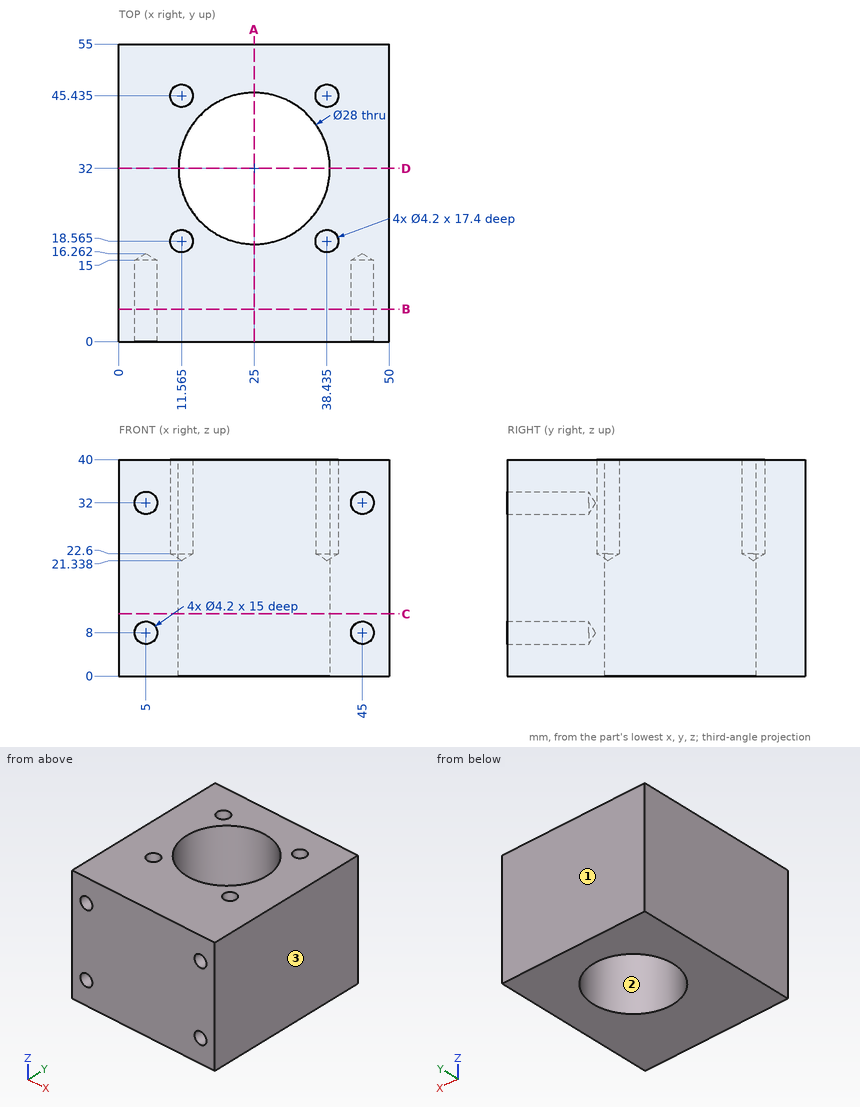
Print and shaded views of the part. All mm, measured from the part's lowest x, y and z. Give positions to 0.01 mm unless a question says otherwise; leave off trailing zeros. Loops run counter-clockwise (first coordinate to the right, second up) from the corner with the lowest first, then second, coordinate; pieces in that order, holes last.
1) Saw through at C-C (z = 11.5). Write the cut outline in (x, y), plus the area to 3 significant figures.
2) Saw through at A-A (x = 25). Write the cut outline in (y, z).
3) Saw through at D-D (y = 32). Write the cut outline in (x, z), plus the area to 3 significant figures.
4) Saw through at B-B (y = 6). Write the cut outline in (x, z), plus the area to 3 significant figures.
5) Wall check: line 1 (Z direction, x = 45, y = 8); line 2 (X direction, y = 17, z = 26) (1 decimal); line 3 (Y direction, x = 12.5, z = 37.5) (1 decimal). Give the ranges that are in metal, low to high.
6) Flat gauge pins, fed straight in: pin 1 Ø4 at (x, z) = (5, 8) entering from -Y; pin 2 Ø3.5 at (x, z) = (5, 32) entering from -Y. Where does each tip first touch, or does it go through?
7) Pull direction X, two halves, no side cores. Call the marked faces 1, 2 and 3: +X half, -X half, draft (parallel to the pull), parting line (faces both ways), or undercut.
Answer block:
1. outline: (0, 0) - (50, 0) - (50, 55) - (0, 55) - close; hole circle Ø28 at (25, 32)
1. area: 2,130 mm2
2. outline: (0, 0) - (18, 0) - (18, 40) - (0, 40) - close; (46, 0) - (55, 0) - (55, 40) - (46, 40) - close
3. outline: (0, 0) - (11, 0) - (11, 40) - (0, 40) - close; (39, 0) - (50, 0) - (50, 40) - (39, 40) - close
3. area: 880 mm2
4. outline: (0, 0) - (50, 0) - (50, 40) - (0, 40) - close; hole circle Ø4.2 at (5, 8); hole circle Ø4.2 at (5, 32); hole circle Ø4.2 at (45, 8); hole circle Ø4.2 at (45, 32)
4. area: 1,940 mm2
5. line 1: z = 0 to 5.9, 10.1 to 29.9, 34.1 to 40
5. line 2: x = 0 to 10.2, 13 to 37, 39.8 to 50
5. line 3: y = 0 to 16.7, 20.4 to 25.7, 38.3 to 43.6, 47.3 to 55
6. pin 1: stops at y = 15.06
6. pin 2: stops at y = 15.21
7. face 1: draft
7. face 2: undercut
7. face 3: +X half
